```python
from build123d import *

# Parameters (mm, degrees)
SKETCH2_R           = 1.5
BOSS_EXTRUDE1_DEPTH = 5


with BuildPart() as part:
    # Sketch2 → Boss-Extrude1 (new body)
    with BuildSketch(Plane.XY):
        with BuildLine():
            Line((807.944636851, 1128.1431403), (807.944636851, 1114.1431403))
            ThreePointArc((807.944636851, 1114.1431403), (803.551238569, 1103.536538582), (792.944636851, 1099.1431403))
            Line((792.944636851, 1099.1431403), (784.694636851, 1099.1431403))
            ThreePointArc((784.694636851, 1099.1431403), (774.088035133, 1094.749742018), (769.694636851, 1084.1431403))
            Line((769.694636851, 1084.1431403), (769.694636851, 1018.1431403))
            ThreePointArc((769.694636851, 1018.1431403), (774.088035133, 1007.536538582), (784.694636851, 1003.1431403))
            Line((784.694636851, 1003.1431403), (891.194636851, 1003.1431403))
            ThreePointArc((891.194636851, 1003.1431403), (901.801238569, 1007.536538582), (906.194636851, 1018.1431403))
            Line((906.194636851, 1018.1431403), (906.194636851, 1084.1431403))
            ThreePointArc((906.194636851, 1084.1431403), (901.801238569, 1094.749742018), (891.194636851, 1099.1431403))
            Line((891.194636851, 1099.1431403), (882.944636851, 1099.1431403))
            ThreePointArc((882.944636851, 1099.1431403), (872.338035133, 1103.536538582), (867.944636851, 1114.1431403))
            Line((867.944636851, 1114.1431403), (867.944636851, 1128.1431403))
            ThreePointArc((867.944636851, 1128.1431403), (863.551238569, 1138.749742018), (852.944636851, 1143.1431403))
            Line((852.944636851, 1143.1431403), (822.944636851, 1143.1431403))
            ThreePointArc((822.944636851, 1143.1431403), (812.338035133, 1138.749742018), (807.944636851, 1128.1431403))
        make_face()
        with Locations((837.944636851, 1119.927749991)):
            Circle(SKETCH2_R, mode=Mode.SUBTRACT)
        with Locations((784.694636851, 1012.8931403)):
            Circle(SKETCH2_R, mode=Mode.SUBTRACT)
        with Locations((886.194636851, 1044.1431403)):
            Circle(SKETCH2_R, mode=Mode.SUBTRACT)
        with Locations((886.194636851, 1058.1431403)):
            Circle(SKETCH2_R, mode=Mode.SUBTRACT)
        with Locations((789.694636851, 1044.1431403)):
            Circle(SKETCH2_R, mode=Mode.SUBTRACT)
        with Locations((789.694636851, 1058.1431403)):
            Circle(SKETCH2_R, mode=Mode.SUBTRACT)
        with Locations((784.694636851, 1089.3931403)):
            Circle(SKETCH2_R, mode=Mode.SUBTRACT)
        with Locations((891.194636851, 1089.3931403)):
            Circle(SKETCH2_R, mode=Mode.SUBTRACT)
        with Locations((891.194636851, 1012.8931403)):
            Circle(SKETCH2_R, mode=Mode.SUBTRACT)
        with BuildLine():
            Line((845.444636851, 1009.1431403), (830.444636851, 1009.1431403))
            ThreePointArc((830.444636851, 1009.1431403), (825.444636851, 1014.1431403), (830.444636851, 1019.1431403))
            Line((830.444636851, 1019.1431403), (845.444636851, 1019.1431403))
            ThreePointArc((845.444636851, 1019.1431403), (850.444636851, 1014.1431403), (845.444636851, 1009.1431403))
        make_face(mode=Mode.SUBTRACT)
    extrude(amount=BOSS_EXTRUDE1_DEPTH)


solid = part.part
```
Design review of the part built by this model. Coordinates are the model's own, in mm. A direction names the side the tool comes from. Give positions to 0.01 mm unless a question says otherwise; leave off trailing zeros. Order: outer loops, then holes, each group sorted by start corner. A loop starts at its lowest first (then second) coordinate and runs counter-clockwise, first axis right, second up. Notation, with made-up numbers: (-8.5, 44) - (5.5, 44) arc R28 ccw to (5.5, 63) - close; hole circle Ø1 at (-36, 11). An arc over 180 degrees is marked (long way). Use a Markdown table: item, result. Add a question column.
(1) Add section A-A on z = 1.9. Give the number of separate pieces and of enclosed holes in the cut face, then the cut area to 3 significant figures.
(2) Add section C-C on x = 815. Give the boundary of the cut face in (y, z).
(3) Clearance check with flat-ended pins moving along their axes: P1, Ø3.5, axis at x = 891.19, y = 1089.39, coming from the -Z side; P2, Ø1.5, axis at x = 873, z = 2, coming from the +Y side; P3, Ø2.5, axis at x = 885.5, z = 3, coming from the +Y side. State where each tip first meets the part, or that it passes through.
(4) Wall thickness on probe 1 along Y at (x, z) = (891.5, 3.7); probe 2 along Y at (x, z) = (790, 1.45); probe 3 along Y at (x, z) = (835, 4.8): over which ranges is each line inside the solid? List them lowest first. Write a range as [from, to].
(5) Machinability: for faces 4 (the face through (906.195, 1051, 2)), 5 (the face through (807.945, 1121, 2)), 6 (the face through (825.446, 1014.033, 2.465)), 7 (the face through (837, 1059, 0)), 8 (the face through (867.945, 1121, 2)), which of the approach directions +Z, -Z, +X, -X, +Y, -Y give a long, thin tool a straight path to every point of the face, cutting with its end or side? Answer none if there is none.
(6) Add section B-B on y = 1109.5. Give the boundary of the cut face in (x, z), then the cut area to 3 significant figures.
(7) Mouldability with a two-part tool opening along X and no side actions: class faces 1 (the face through (838, 1009.143, 2)), 2 (the face through (863.7, 1138.6, 2.5)), 3 (the face through (887, 1099.143, 2)) as +X half, -X half, draft (parallel to the pull), parting line (faces both ways), or undercut.
Report:
| question | item | result |
|---|---|---|
| 1 | separate pieces | 1 |
| 1 | enclosed holes | 10 |
| 1 | area | 15,300 mm² |
| 2 | outline | (1003.14, 0) - (1140.87, 0) - (1140.87, 5) - (1003.14, 5) - close |
| 3 | P1 | stops at z = 0 |
| 3 | P2 | stops at y = 1103.63 |
| 3 | P3 | stops at y = 1099.14 |
| 4 | probe 1 | y = [1003.15, 1011.42], [1014.36, 1087.92], [1090.86, 1099.14] |
| 4 | probe 2 | y = [1003.14, 1042.67], [1045.61, 1056.67], [1059.61, 1099.14] |
| 4 | probe 3 | y = [1003.14, 1009.14], [1019.14, 1143.14] |
| 5 | face 4 | +Z, -Z, +X, +Y, -Y |
| 5 | face 5 | +Z, -Z, -X, +Y |
| 5 | face 6 | +Z, -Z |
| 5 | face 7 | -Z, +X, -X, +Y, -Y |
| 5 | face 8 | +Z, -Z, +X, +Y |
| 6 | outline | (807.21, 0) - (868.68, 0) - (868.68, 5) - (807.21, 5) - close |
| 6 | area | 307 mm² |
| 7 | face 1 | undercut |
| 7 | face 2 | +X half |
| 7 | face 3 | draft |
